Source: three-view drawing plus pictorial views. Frame: mm from the lowest corner of the part. A direction names the side the tool comes from. Give positions to 0.01 mm unless a question says otherwise; leave off trailing zeros. Write each loop counter-clockwise with the first axis right and the second up, starting at its lowest first coordinate (ties: lowest second). Pieces come first, ordered by that corner, then holes.
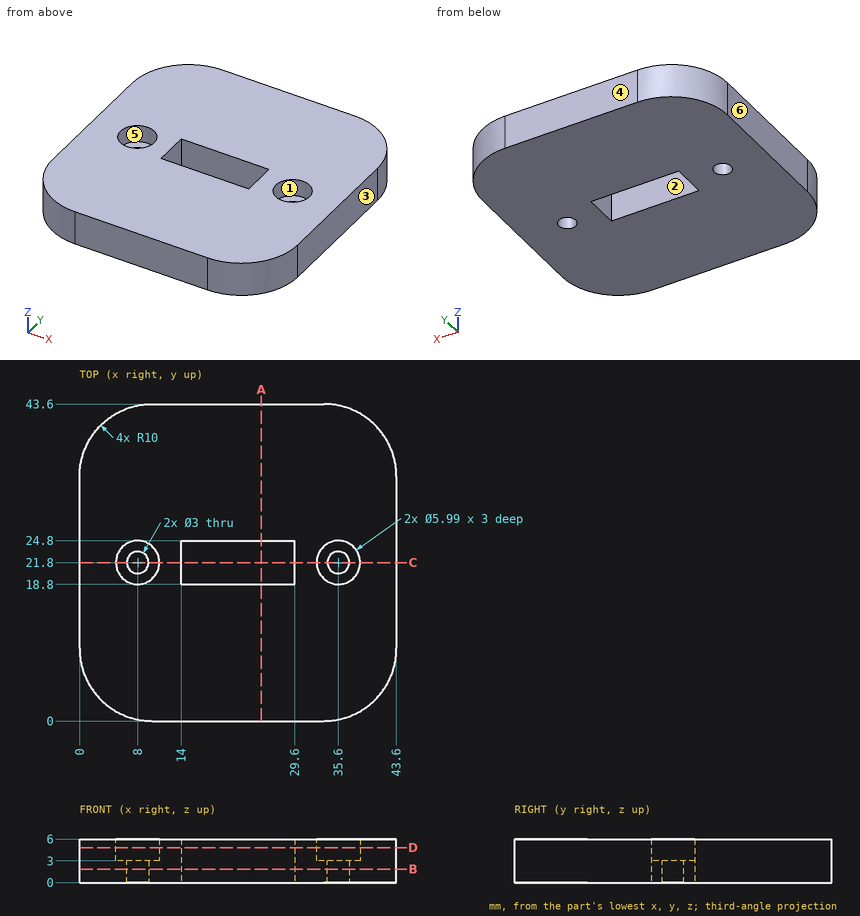
Q1. Section C-C on y = 21.8. Output: boundary loops of the cut face in (x, z) (3 decimals), plus the area to 3 significant figures.
Filled sheet:
outline: (0, 0) - (6.5, 0) - (6.5, 3) - (5.005, 3) - (5.005, 6) - (0, 6) - close; (9.5, 0) - (14, 0) - (14, 6) - (10.995, 6) - (10.995, 3) - (9.5, 3) - close; (29.6, 0) - (34.1, 0) - (34.1, 3) - (32.605, 3) - (32.605, 6) - (29.6, 6) - close; (37.1, 0) - (43.6, 0) - (43.6, 6) - (38.595, 6) - (38.595, 3) - (37.1, 3) - close
area: 114 mm2
Q2. Access query for the marked faces 1, 2 and 3. Directions: +Z, -Z, +X, -X, +Y, -Y. A direction counts if a zero-diameter tool reaches every point of the face in a straight line with its end or side. Return the directions, or none.
Filled sheet:
face 1: +Z
face 2: +Z, -Z
face 3: +Z, -Z, +X, +Y, -Y
Q3. Ray query, line 1 along X through (y, z) = (19.5, 4.2); line 2 along Y through (x, z) = (27, 1.85); line 3 along Y through (x, z) = (35.6, 2.05). Return the intervals inside material, ascending.
Filled sheet:
line 1: x = 0 to 6.08, 9.92 to 14, 29.6 to 33.68, 37.52 to 43.6
line 2: y = 0 to 18.8, 24.8 to 43.6
line 3: y = 0.2 to 20.3, 23.3 to 43.4
Q4. Pull-direction query (X, two-part tool) for the marked faces 4, 5 and 6; classes: released by +X, released by -X, zero draft, split by the parting line, or undercut.
Filled sheet:
face 4: zero draft
face 5: undercut
face 6: released by -X
Q5. Section A-A on x = 25. Output: boundary loops of the cut face in (y, z).
Filled sheet:
outline: (0, 0) - (18.8, 0) - (18.8, 6) - (0, 6) - close; (24.8, 0) - (43.6, 0) - (43.6, 6) - (24.8, 6) - close
Q6. Pin query (flat end, axial travel): P1, Ø2.5, axis at x = 8, y = 21.8, coming from the +Z side; P2, Ø1.8, axis at x = 35, y = 21.5, coming from the +Z side. Return the tip coordinate at first contact, or that it passes through.
Filled sheet:
P1: passes through
P2: stops at z = 3
Q7. Section D-D on z = 4.8. Output: boundary loops of the cut face in (x, y) (3 decimals).
Filled sheet:
outline: (0, 10) arc R10 ccw to (10, 0) - (33.6, 0) arc R10 ccw to (43.6, 10) - (43.6, 33.6) arc R10 ccw to (33.6, 43.6) - (10, 43.6) arc R10 ccw to (0, 33.6) - close; hole circle Ø5.99 at (8, 21.8); hole (14, 18.8) - (29.6, 18.8) - (29.6, 24.8) - (14, 24.8) - close; hole circle Ø5.99 at (35.6, 21.8)
Q8. Section B-B on z = 1.85. Output: boundary loops of the cut face in (x, y), plus the area to 3 significant figures.
Filled sheet:
outline: (0, 10) arc R10 ccw to (10, 0) - (33.6, 0) arc R10 ccw to (43.6, 10) - (43.6, 33.6) arc R10 ccw to (33.6, 43.6) - (10, 43.6) arc R10 ccw to (0, 33.6) - close; hole circle Ø3 at (8, 21.8); hole (14, 18.8) - (29.6, 18.8) - (29.6, 24.8) - (14, 24.8) - close; hole circle Ø3 at (35.6, 21.8)
area: 1,710 mm2
